The drawing under review shows one solid part. Ordinate dimensions are in mm from its lowest x, y, z. A direction names the side the tool comes from. Coordinates: 2 decimals unless noted, no trailing zeros. Loops run counter-clockwise (first coordinate to the right, second up) from the corner with the lowest first, then second, coordinate; pieces in that order, holes last. Notation, with made-up numbers: M -15,49 L 23,49 A11 cw 23,62 Z; hole C 56.25,-20 d8. An arc over 180 degrees is marked long. Use one line per item in the form item = value.
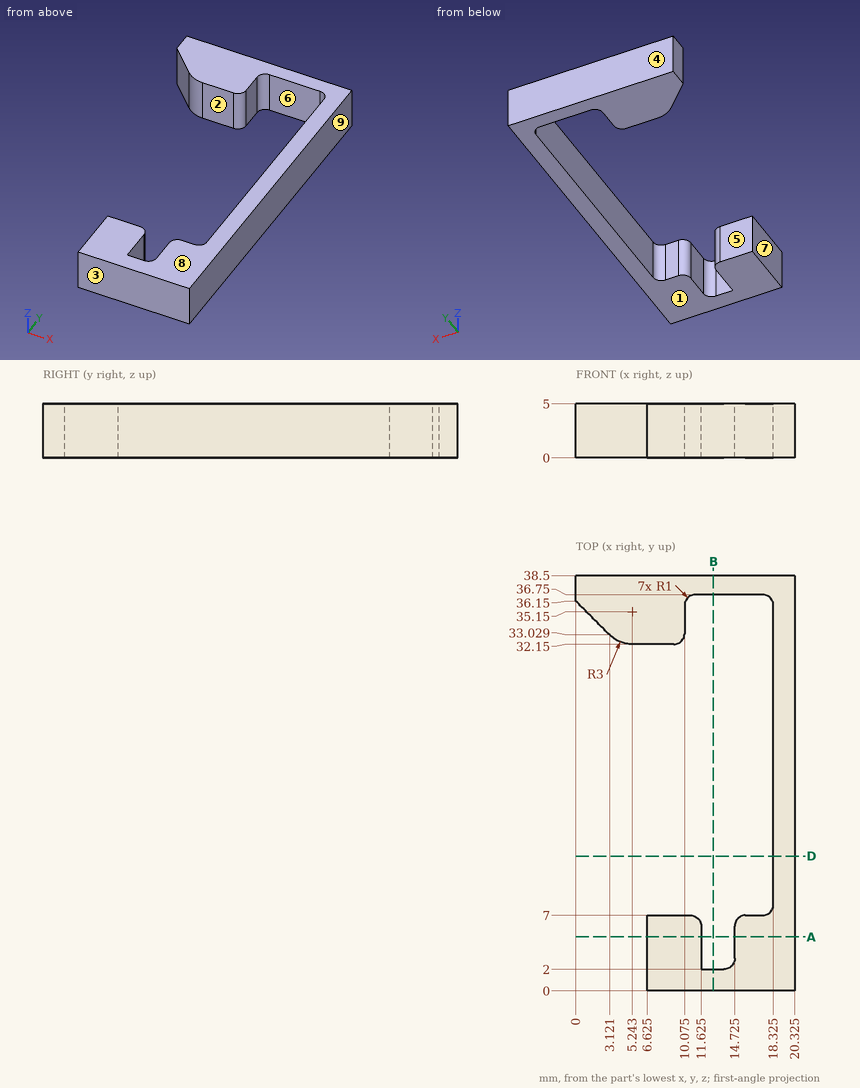
1. For pin 1 Ø1.5 at (y, z) = (16.5, 2) entering from -X (1 decimal); pin 2 Ø1.5 at (y, z) = (4.5, 3.5) entering from -X (1 decimal), all flat-tipped, find the tip position at first contact; note any pin that passes through.
Computed values:
pin_1 = 18.3
pin_2 = 6.6
2. Tool access review of the marked faces 5, 6, 7, 8 and 9: name each direction out of +Z, -Z, +X, -X, +Y, -Y from which nothing blocks a thin tool from reaching the whole face with its end or side.
Computed values:
face_5 = +Z, -Z, -X
face_6 = +Z, -Z
face_7 = +Z, -Z, -X, -Y
face_8 = +Z, +X, -X, +Y, -Y
face_9 = +Z, -Z, +X, +Y, -Y
3. Draft analysis for pull direction Y (two halves, no side actions). For the marked faces 1, 2, 3 and 4, state which applies: +Y half, -Y half, draft (parallel to the pull), parting line (faces both ways), or undercut.
Computed values:
face_1 = draft
face_2 = undercut
face_3 = -Y half
face_4 = +Y half
4. Consider section B-B on x = 12.75. Write out the cut boundary in (y, z).
Computed values:
outline = M 0,0 L 2,0 L 2,5 L 0,5 Z; M 36.75,0 L 38.5,0 L 38.5,5 L 36.75,5 Z
5. Wall thickness on line 1 along Y through (x, z) = (17, 2.8); line 2 along Y through (x, z) = (8, 2.4); line 3 along X through (y, z) = (25, 3.1) (1 decimal): over which ranges is each line inside the solid? List them lowest first. Write a range as from..to.
Computed values:
line_1 = 0..7, 36.75..38.5
line_2 = 0..7, 32.15..38.5
line_3 = 18.3..20.3
6. Consider section A-A on y = 5. Write out the cut boundary in (x, z) (1 decimal), plus the area to 3 significant figures.
Computed values:
outline = M 6.6,0 L 11.6,0 L 11.6,5 L 6.6,5 Z; M 14.7,0 L 20.3,0 L 20.3,5 L 14.7,5 Z
area = 53.0 mm2
7. Consider section D-D on y = 12.5. Write out the cut boundary in (x, z) (1 decimal), plus the area to 3 significant figures.
Computed values:
outline = M 18.3,0 L 20.3,0 L 20.3,5 L 18.3,5 Z
area = 10.0 mm2
